For this review, take the finished solid that the model builds, in its own axes (mm). Face numbers are marked on the shaded views. Give positions to 0.01 mm unless a question says otherwise; leave off trailing zeros. Loops run counter-clockwise (first coordinate to the right, second up) from the corner with the lowest first, then second, coordinate; pieces in that order, holes last.
```python
from build123d import *

# Parameters (mm, degrees)
F1_DEPTH = 25
F3_D     = 3.3
F3_DEPTH = 2
F3_TIP   = 0.9914200214


with BuildPart() as f1:
    # F0 (on Top) → F1 (new body)
    with BuildSketch(Plane.XY):
        with BuildLine():
            Line((-4.6761400443, -1.6786290068), (4.6761400443, -1.6786290068))
            ThreePointArc((4.6761400443, -1.6786290068), (0, 8.9213709932), (-4.6761400443, -1.6786290068))
        make_face()
        with BuildLine():
            Line((3.8, 0.1213709932), (-3.8, 0.1213709932))
            ThreePointArc((-3.8, 0.1213709932), (0, 7.1213709932), (3.8, 0.1213709932))
        make_face(mode=Mode.SUBTRACT)
    extrude(amount=F1_DEPTH)

    # F3
    with Locations(Plane.XZ.offset(1.6786290068)):
        with Locations((0, 12.5)):
            Hole(F3_D / 2, depth=F3_DEPTH)
            with Locations((0, 0, -(F3_DEPTH + F3_TIP / 2))):  # 118° drill point
                Cone(0, F3_D / 2, F3_TIP, mode=Mode.SUBTRACT)


solid = f1.part
```
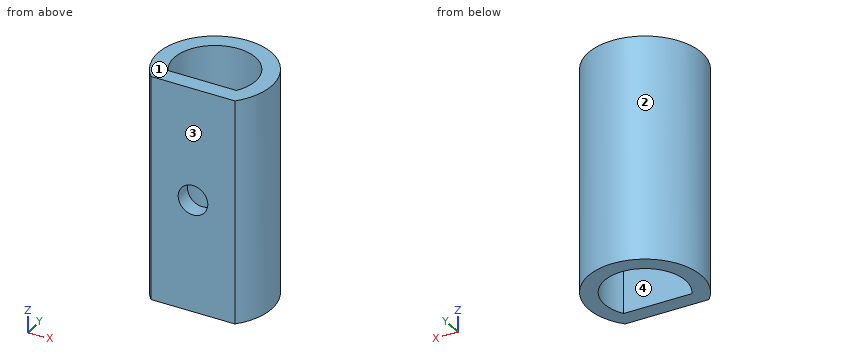
Q1. For pin 1 Ø5 at (x, z) = (4.5, 18) entering from +Y; pin 2 Ø4 at (x, z) = (-0.5, 6.5) entering from +Y; pin 3 Ø2 at (x, z) = (0, 12.5) entering from -Y; pin 4 Ø1.5 at (x, z) = (-4.5, 12) entering from +Y, all flat-tipped, find the tip position at first contact; note any pin that passes through.
Answers:
pin 1: stops at y = 8.6
pin 2: stops at y = 8.92
pin 3: stops at y = 7.01
pin 4: stops at y = 7.69
Q2. Consider section D-D on x = 3.5. Give the boundary of the cut face in (y, z).
Answers:
outline: (-1.68, 0) - (0.12, 0) - (0.12, 25) - (-1.68, 25) - close; (5.47, 0) - (7.87, 0) - (7.87, 25) - (5.47, 25) - close
Q3. Consider section B-B on x = 0. Give the boundary of the cut face in (y, z).
Answers:
outline: (-1.68, 0) - (0.12, 0) - (0.12, 10.85) - (-1.68, 10.85) - close; (-1.68, 14.15) - (0.12, 14.15) - (0.12, 25) - (-1.68, 25) - close; (7.12, 0) - (8.92, 0) - (8.92, 25) - (7.12, 25) - close
Q4. Consider section C-C on z = 12.5. Give the boundary of the cut face in (x, y).
Answers:
outline: (-4.68, -1.68) - (-1.65, -1.68) - (-1.65, 0.12) - (-3.8, 0.12) arc R4.53 cw (long way) to (3.8, 0.12) - (1.65, 0.12) - (1.65, -1.68) - (4.68, -1.68) arc R6.33 ccw (long way) to start
Q5. For probe 1 along Y at (x, z) = (0, 16.75); probe 2 along Z at (x, y) = (0, -0.65); probe 3 along X at (y, z) = (1.5, 8.25), list the stretches that pass through material, from the lowest coordinate up.
Answers:
probe 1: y = -1.68 to 0.12, 7.12 to 8.92
probe 2: z = 0 to 10.85, 14.15 to 25
probe 3: x = -6.24 to -4.4, 4.4 to 6.24
Q6. Consider section A-A on y = 1.25. Give the boundary of the cut face in (x, z), plus the area to 3 significant figures.
Answers:
outline: (-6.19, 0) - (-4.33, 0) - (-4.33, 25) - (-6.19, 25) - close; (4.33, 0) - (6.19, 0) - (6.19, 25) - (4.33, 25) - close
area: 93.0 mm2
Q7. Mouldability with a two-part tool opening along Y and no side actions: class the marked faces 1, 2, 3 and 4 as +Y half, -Y half, draft (parallel to the pull), parting line (faces both ways), or undercut.
Answers:
face 1: draft
face 2: parting line
face 3: -Y half
face 4: undercut
